from build123d import *

# Parameters (mm, degrees)
CROQUIS1_R                 = 10
CROQUIS1_R_2               = 6.25
SALIENTE_EXTRUIR1_DEPTH    = 13
SALIENTE_EXTRUIR2_START    = -30
CROQUIS2_R                 = 10
CROQUIS2_R_2               = 7.48
SALIENTE_EXTRUIR2_DEPTH    = 30
CORTAR_EXTRUIR1_DEPTH      = 39.57274278
CORTAR_EXTRUIR1_DEPTH_BACK = 39.57274278
CROQUIS3_R                 = 2.5


with BuildPart() as part:
    # Croquis1 → Saliente-Extruir1 (new body)
    with BuildSketch(Plane.XY):
        with Locations(Location((-9.736276302, -4.083177315, 0), (0, 0, 180))):
            Circle(CROQUIS1_R)
        with Locations(Location((-9.736276302, -4.083177315, 0), (0, 0, 180))):
            Circle(CROQUIS1_R_2, mode=Mode.SUBTRACT)
    extrude(amount=SALIENTE_EXTRUIR1_DEPTH)

    # Croquis2 → Saliente-Extruir2 (add)
    with BuildSketch(Plane.XY.offset(SALIENTE_EXTRUIR2_START)):
        with Locations(Location((-9.736276302, -4.083177315, 0), (0, 0, 180))):
            Circle(CROQUIS2_R)
        with Locations((-9.736276302, -4.083177315)):
            Circle(CROQUIS2_R_2, mode=Mode.SUBTRACT)
    extrude(amount=SALIENTE_EXTRUIR2_DEPTH)

    # Croquis3 → Cortar-Extruir1 (cut, two sides: drawn at the far end of the back side and taken through both)
    with BuildSketch(Plane(origin=(0, 0, 0), x_dir=(1, 0, 0), z_dir=(0, 1, 0)).offset(-CORTAR_EXTRUIR1_DEPTH_BACK)):
        with Locations(Location((-9.736276302, 15, 0), (0, 0, 270))):
            Circle(CROQUIS3_R)
        with Locations(Location((-9.736276302, 2, 0), (0, 0, 270))):
            Circle(CROQUIS3_R)
    extrude(amount=CORTAR_EXTRUIR1_DEPTH + CORTAR_EXTRUIR1_DEPTH_BACK, mode=Mode.SUBTRACT)


solid = part.part
The model under review builds one solid part; all positions refer to its coordinate system, in mm. A direction names the side the tool comes from. Coordinates: 2 decimals unless noted, no trailing zeros. Write each loop counter-clockwise with the first axis right and the second up, starting at its lowest first coordinate (ties: lowest second). Pieces come first, ordered by that corner, then holes. Notation, with made-up numbers: (30.5, 30.25) - (55.5, 30.25) arc R30 cw to (55.5, 61.25) - close; hole circle Ø10 at (73.5, 32.25). An arc over 180 degrees is marked (long way). Answer as a JSON object with one key per item and string values. Group by question number.
1. Mouldability with a two-part tool opening along Y and no side actions: class faces 3 (the face through (-14.35, 4.79, -8.8)), 4 (the face through (-14, -9, 13)), 5 (the face through (-2.6, -1.84, -15.21)) as pulls with the +Y half, pulls with the -Y half, needs draft (parallel to the pull), parting line crosses it, or undercut.
2. Add section A-A (y = 0.75). Give the boundary of the cut face in (x, z), plus the area to 3 significant figures.
3. Clearance check with flat-ended pins moving along their axes: pin 1 Ø6 at (y, z) = (-7.5, -17.5) entering from -X; pin 2 Ø12 at (x, z) = (-16.5, -19.5) entering from -Y; pin 3 Ø3 at (x, z) = (-11, -2) entering from +Y. State where each tip first meets the part, or that it passes through.
4. Add section B-B (z = -16). Give the boundary of the cut face in (x, y).
5. Add section C-C (x = -6). Give the boundary of the cut face in (y, z), plus the area to 3 significant figures.
6. To check wall thickness, follow probe 1 along X at (y, z) = (-12, -15); probe 2 along Y at (x, z) = (-15.25, -3); probe 3 along X at (y, z) = (-3.75, -20). State the ranges of each line that lie inside material, in increasing order.
7. Add section D-D (y = 4). Give the boundary of the cut face in (x, z).
8. Machinability: for faces 1 (the face through (-15.698, -5.961, 6.409)), 2 (the face through (-3, -4, 0)), which of the approach directions +Z, -Z, +X, -X, +Y, -Y give a long, thin tool a straight path to every point of the face, cutting with its end or side? Answer none if there is none.
Findings:
{
 "1": {"face 3": "parting line crosses it", "face 4": "needs draft", "face 5": "undercut"},
 "2": {"outline": "(-18.49, -30) - (-15.45, -30) - (-15.45, 0) - (-13.7, 0) - (-13.7, 13) - (-18.49, 13) - close; (-5.77, 0) - (-4.03, 0) - (-4.03, -30) - (-0.98, -30) - (-0.98, 13) - (-5.77, 13) - close", "area": "307 mm²"},
 "3": {"pin 1": "x = -19.73", "pin 2": "y = -14.05", "pin 3": "y = 5.67"},
 "4": {"outline": "(-12.03, -13.82) - (-12.03, -11.2) arc R7.48 cw to (-12.03, 3.04) - (-12.03, 5.65) arc R10 ccw to start; (-7.44, -13.82) arc R10 ccw to (-7.44, 5.65) - (-7.44, 3.04) arc R7.48 cw to (-7.44, -11.2) - close"},
 "5": {"outline": "(-13.36, -30) - (-10.56, -30) - (-10.56, 0) - (-9.09, 0) - (-9.09, 13) - (-13.36, 13) - close; (0.93, 0) - (2.4, 0) - (2.4, -30) - (5.19, -30) - (5.19, 13) - (0.93, 13) - close", "area": "279 mm²"},
 "6": {"probe 1": "-15.85 to -12.24, -7.24 to -3.63", "probe 2": "-12.43 to -9.14, 0.97 to 4.26", "probe 3": "-19.73 to -17.21, -2.26 to 0.26"},
 "7": {"outline": "(-15.62, -30) - (-3.85, -30) - (-3.85, 13) - (-15.62, 13) - close; hole circle Ø5 at (-9.74, -15); hole circle Ø5 at (-9.74, -2)"},
 "8": {"face 1": "+Z, -Z", "face 2": "-Z"}
}
